from build123d import *

# Parameters (mm, degrees)
BOSS_EXTRUDE1_DEPTH                                 = 9
BOSS_EXTRUDE1_DEPTH_BACK                            = 1
CUT_EXTRUDE1_DEPTH                                  = 3
CSK_FOR_M4_COUNTERSUNK_FLAT_HEAD_SCREW2_D           = 4.5
CSK_FOR_M4_COUNTERSUNK_FLAT_HEAD_SCREW2_CSINK_D     = 8.5
CSK_FOR_M4_COUNTERSUNK_FLAT_HEAD_SCREW2_CSINK_ANGLE = 90
FILLET1_R                                           = 15
FILLET2_R                                           = 10
FILLET3_R                                           = 3
SKETCH12_R                                          = 1.65
CUT_EXTRUDE2_DEPTH                                  = 181.248579312


with BuildPart() as part:
    # Sketch1 → Boss-Extrude1 (new, two sides: drawn at the far end of the back side and taken through both)
    with BuildSketch(Plane.XY.offset(-BOSS_EXTRUDE1_DEPTH_BACK)):
        Polygon((-14.65789802, 119.616999761), (13.633055873, 119.616999761), (13.633055873, 139.616999761), (13.633055873, 158.176865611), (17.633055873, 165.105068841), (-6.615655433, 179.105068841), (-10.615655433, 172.176865611), (-14.65789802, 165.175496074), (-14.65789802, 158.176865611), (-14.65789802, 139.616999761), align=None)
    extrude(amount=BOSS_EXTRUDE1_DEPTH + BOSS_EXTRUDE1_DEPTH_BACK)

    # Sketch3 → Cut-Extrude1 (cut)
    with BuildSketch(Plane(origin=(0, 0, -1), x_dir=(-1, 0, 0), z_dir=(0, 0, -1))):
        with BuildLine():
            Line((-15, 144.248115566), (-15, 114.785930714))
            Line((-15, 114.785930714), (15, 114.785930714))
            Line((15, 114.785930714), (15, 144.248115566))
            ThreePointArc((15, 144.248115566), (0, 145), (-15, 144.248115566))
        make_face()
    extrude(amount=-CUT_EXTRUDE1_DEPTH, mode=Mode.SUBTRACT)

    # CSK for M4 Countersunk Flat Head Screw2 (through all)
    with Locations(Plane.XY.offset(9)):
        with Locations((0, 0), (8, 136.785930714), (-8, 136.785930714), (0, 124.785930714)):
            CounterSinkHole(CSK_FOR_M4_COUNTERSUNK_FLAT_HEAD_SCREW2_D / 2, CSK_FOR_M4_COUNTERSUNK_FLAT_HEAD_SCREW2_CSINK_D / 2, counter_sink_angle=CSK_FOR_M4_COUNTERSUNK_FLAT_HEAD_SCREW2_CSINK_ANGLE)

    # Fillet1
    fillet1_edges = [part.edges().sort_by_distance(p)[0] for p in [
        (-14.65789802, 165.175496074, 4),
        (13.633055873, 158.176865611, 4),
    ]]
    fillet(fillet1_edges, radius=FILLET1_R)

    # Fillet2
    fillet2_edges = [part.edges().sort_by_distance(p)[0] for p in [
        (13.633055873, 119.616999761, 5.5),
        (-14.65789802, 119.616999761, 5.5),
    ]]
    fillet(fillet2_edges, radius=FILLET2_R)

    # Fillet3
    fillet3_edges = [part.edges().sort_by_distance(p)[0] for p in [
        (-14.65789802, 144.282102161, 0.5),
        (13.633055873, 144.379181239, 0.5),
    ]]
    fillet(fillet3_edges, radius=FILLET3_R)

    # Sketch12 → Cut-Extrude2 (cut, through all)
    with BuildSketch(Plane(origin=(0, 0, -1), x_dir=(-1, 0, 0), z_dir=(0, 0, -1))):
        with Locations((4.49129978, 172.105068841)):
            Circle(SKETCH12_R)
        with Locations((-9.633055873, 165.105068841)):
            Circle(SKETCH12_R)
        with Locations((0.146785414, 163.038543864)):
            Circle(SKETCH12_R)
    extrude(amount=-CUT_EXTRUDE2_DEPTH, mode=Mode.SUBTRACT)


solid = part.part
Could you check a few things on this model? Use its own coordinates, in mm. A direction names the side the tool comes from. Give positions to 0.01 mm unless a question says otherwise; leave off trailing zeros. Write each loop counter-clockwise with the first axis right and the second up, starting at its lowest first coordinate (ties: lowest second). Pieces come first, ordered by that corner, then holes. Notation, with made-up numbers: (-7, 81) -> (-2, 81) arc R14 cw to (-2, 92) -> close; hole circle Ø4 at (56.25, 0). An arc over 180 degrees is marked (long way). Answer as CSV lines item,"result". Start each with the question number.
(1) If we section it at D-D, the plane x = -8: Write out the boundary of the cut face in (y, z).
(2) I'm going to push flat-ended pins straight in: pin 1 Ø6 at (x, y) = (8, 136.79) entering from -Z; pin 2 Ø1.5 at (x, z) = (-5, 6.5) entering from +Y. Where does each tip first touch, or does it pass through?
(3) Please list where these lines run through material, in increasing order: line 1 (Y direction, x = 0.5, z = 4); line 2 (X direction, y = 132, z = 3.5); line 3 (Z direction, x = -2.5, y = 142).
(4) If we section it at B-B, the plane y = 171.5: Write out the boundary of the cut face in (x, z), and give its area (3 significant figures).
(5) If we mould it in two halves opening along Y, with no side actions, what happens to faces 1 (the face through (-14.658, 146, 5)), 2 (the face through (16.624, 163.357, 3.93)), 3 (the face through (-7.707, 139.017, 4.465)), 4 (the face through (9.85, 166.74, 3.93))? For each: +Y half, -Y half, draft (parallel to the pull), parting line (faces both ways), or undercut.
(6) If we section it at A-A, the plane x = 0: Write out the boundary of the cut face in (y, z).
(7) Which directions (+Z, -Z, +X, -X, +Y, -Y) give clear straight access to the entire face, cutting with the end or side of a thin tool? Please do faces 5 (the face through (-0.7, 145, 0.5)), 6 (the face through (0.293, 127.017, 4.465)).
(8) If we section it at C-C, the plane z = 8.25: Write out the boundary of the cut face in (x, y), and give its area (3 significant figures).
Answer list:
1,outline,"(120.19, 2) -> (134.54, 2) -> (134.54, 7) -> (132.54, 9) -> (120.19, 9) -> close; (139.04, 2) -> (144.79, 2) -> (144.79, -1) -> (176.71, -1) -> (176.71, 9) -> (141.04, 9) -> (139.04, 7) -> close"
2,pin 1,"z = 2"
2,pin 2,"y = 178.61"
3,line 1,"119.62 to 122.59, 126.98 to 161.52, 164.56 to 175"
3,line 2,"-14.66 to 13.63"
3,line 3,"2 to 9"
4,outline,"(-11.01, -1) -> (-6.03, -1) -> (-6.03, 9) -> (-11.01, 9) -> close; (-2.96, -1) -> (6.56, -1) -> (6.56, 9) -> (-2.96, 9) -> close"
4,area,"145 mm^2"
5,face 1,"draft"
5,face 2,"-Y half"
5,face 3,"undercut"
5,face 4,"undercut"
6,outline,"(119.62, 2) -> (122.54, 2) -> (122.54, 7) -> (120.54, 9) -> (119.62, 9) -> close; (127.04, 2) -> (145, 2) -> (145, -1) -> (161.4, -1) -> (161.4, 9) -> (129.04, 9) -> (127.04, 7) -> close; (164.68, -1) -> (175.29, -1) -> (175.29, 9) -> (164.68, 9) -> close"
7,face 5,"-Z, -Y"
7,face 6,"+Z, -Z"
8,outline,"(-14.66, 129.62) arc R10 ccw to (-4.66, 119.62) -> (3.63, 119.62) arc R10 ccw to (13.63, 129.62) -> (13.63, 154.16) arc R15 cw to (15.64, 161.66) -> (17.63, 165.11) -> (-6.62, 179.11) -> (-12.65, 168.66) arc R15 ccw to (-14.66, 161.16) -> close; hole circle Ø7 at (-8, 136.79); hole circle Ø3.3 at (-4.49, 172.11); hole circle Ø7 at (0, 124.79); hole circle Ø3.3 at (-0.15, 163.04); hole circle Ø7 at (8, 136.79); hole circle Ø3.3 at (9.63, 165.11)"
8,area,"1,340 mm^2"
